Could you check a few things on this drawing? It's one solid part, dimensions in mm from its lowest x, y, z. Round coordinates to 2 decimals unless told otherwise and drop trailing zeros. Loops run counter-clockwise (first coordinate to the right, second up) from the corner with the lowest first, then second, coordinate; pieces in that order, holes last. Notation, with made-up numbers: M 49.25,37.25 L 82.25,37.25 A19 cw 82.25,59.25 Z; hole C -35,-4.75 d6. An arc over 180 degrees is marked long. Return JSON: item names as keys, results as strings.
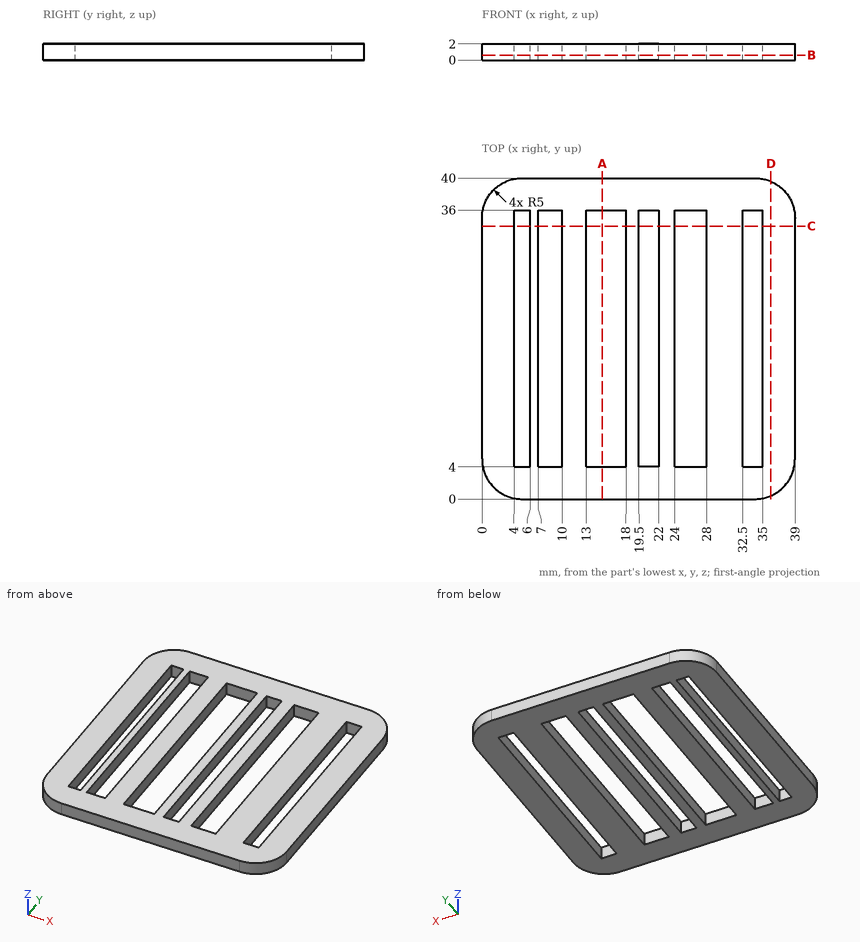
Q1. Suppose I cut it at B-B, the plane z = 0.6. State how many separate pieces and enclosed holes the cut face has, plus the area to 3 significant figures.
Results:
{"separate pieces": "1", "enclosed holes": "6", "area": "931 mm2"}
Q2. Suppose I cut it at D-D, the plane x = 36. Please give me the cut outline in (y, z).
Results:
{"outline": "M 0.42,0 L 39.58,0 L 39.58,2 L 0.42,2 Z"}
Q3. Suppose I cut it at A-A, the plane x = 15. Please give me the cut outline in (y, z), plus the area to 3 significant figures.
Results:
{"outline": "M 0,0 L 4,0 L 4,2 L 0,2 Z; M 36,0 L 40,0 L 40,2 L 36,2 Z", "area": "16.0 mm2"}
Q4. If I drill on line 1 along Y through (x, z) = (21, 0.3); line 2 along X through (y, z) = (2, 0.4); line 3 along X through (y, z) = (36.5, 0.5), over which ranges is the centre line in solid material (lowest first)?
Results:
{"line 1": "y = 0 to 4, 36 to 40", "line 2": "x = 1 to 38", "line 3": "x = 0.23 to 38.77"}
Q5. Suppose I cut it at C-C, the plane y = 34. Please give me the cut outline in (x, z), plus the area to 3 significant figures.
Results:
{"outline": "M 0,0 L 4,0 L 4,2 L 0,2 Z; M 6,0 L 7,0 L 7,2 L 6,2 Z; M 10,0 L 13,0 L 13,2 L 10,2 Z; M 18,0 L 19.5,0 L 19.5,2 L 18,2 Z; M 22,0 L 24,0 L 24,2 L 22,2 Z; M 28,0 L 32.5,0 L 32.5,2 L 28,2 Z; M 35,0 L 39,0 L 39,2 L 35,2 Z", "area": "40.0 mm2"}
